```python
from build123d import *

# Parameters (mm, degrees)
SKETCH1_W           = 100
SKETCH1_H           = 110
BOSS_EXTRUDE1_DEPTH = 1.5
CUT_EXTRUDE1_DEPTH  = 10
FILLET1_R           = 4
SKETCH4_R           = 1.6
CUT_EXTRUDE2_DEPTH  = 10


with BuildPart() as part:
    # Sketch1 → Boss-Extrude1 (new body)
    with BuildSketch(Plane(origin=(0, 0, 0), x_dir=(1, 0, 0), z_dir=(0, 1, 0))):
        Rectangle(SKETCH1_W, SKETCH1_H)
    extrude(amount=BOSS_EXTRUDE1_DEPTH)

    # Sketch2 → Cut-Extrude1 (cut)
    with BuildSketch(Plane(origin=(0, 0, 0), x_dir=(-1, 0, 0), z_dir=(0, -1, 0))):
        Polygon((0, 55), (-24, 55), (-24, 3), (24, 3), (24, 55), align=None)
    extrude(amount=-CUT_EXTRUDE1_DEPTH, mode=Mode.SUBTRACT)

    # Fillet1
    fillet1_edges = [part.edges().sort_by_distance(p)[0] for p in [
        (-24, 0.75, -55),
        (-24, 0.75, -3),
        (24, 0.75, -3),
        (24, 0.75, -55),
        (50, 0.75, 55),
        (-50, 0.75, 55),
        (-50, 0.75, -55),
        (50, 0.75, -55),
    ]]
    fillet(fillet1_edges, radius=FILLET1_R)

    # Sketch4 → Cut-Extrude2 (cut)
    with BuildSketch(Plane(origin=(0, 0, 0), x_dir=(-1, 0, 0), z_dir=(0, -1, 0))):
        with Locations((46, -51)):
            Circle(SKETCH4_R)
        with Locations((46, 51)):
            Circle(SKETCH4_R)
        with Locations((-46, 51)):
            Circle(SKETCH4_R)
        with Locations((-46, -51)):
            Circle(SKETCH4_R)
    extrude(amount=-CUT_EXTRUDE2_DEPTH, mode=Mode.SUBTRACT)


solid = part.part
```
Design review of the part built by this model. Coordinates are the model's own, in mm. A direction names the side the tool comes from. Give positions to 0.01 mm unless a question says otherwise; leave off trailing zeros. Write each loop counter-clockwise with the first axis right and the second up, starting at its lowest first coordinate (ties: lowest second). Pieces come first, ordered by that corner, then holes.
(1) Clearance check with a flat-ended pin moving along its axis: pin 1 Ø0.8 at (x, y) = (0.5, 0.5) entering from -Z. State where the tip first meets the part, or that it passes through.
Checked values:
pin 1: stops at z = -3
(2) Add section A-A (z = -25). Give the boundary of the cut face in (x, y).
Checked values:
outline: (-50, 0) - (-24, 0) - (-24, 1.5) - (-50, 1.5) - close; (24, 0) - (50, 0) - (50, 1.5) - (24, 1.5) - close
(3) Mouldability with a two-part tool opening along X and no side actions: class faces 1 (the face through (25.141, 0.76, -53.797)), 2 (the face through (-48.859, 0.76, 53.797)), 3 (the face through (-1, 1.5, 11)), 4 (the face through (48.859, 0.76, -53.797)) as +X half, -X half, draft (parallel to the pull), parting line (faces both ways), or undercut.
Checked values:
face 1: undercut
face 2: -X half
face 3: draft
face 4: +X half
(4) Add section C-C (x = -21.5). Give the boundary of the cut face in (y, z), and give its area (3 significant figures).
Checked values:
outline: (0, -3.29) - (1.5, -3.29) - (1.5, 55) - (0, 55) - close
area: 87.4 mm2
(5) Add section B-B (y = 0.6). Give the boundary of the cut face in (x, z).
Checked values:
outline: (-50, -51) arc R4 ccw to (-46, -55) - (-28, -55) arc R4 ccw to (-24, -51) - (-24, -7) arc R4 cw to (-20, -3) - (20, -3) arc R4 cw to (24, -7) - (24, -51) arc R4 ccw to (28, -55) - (46, -55) arc R4 ccw to (50, -51) - (50, 51) arc R4 ccw to (46, 55) - (-46, 55) arc R4 ccw to (-50, 51) - close; hole circle Ø3.2 at (-46, -51); hole circle Ø3.2 at (-46, 51); hole circle Ø3.2 at (46, -51); hole circle Ø3.2 at (46, 51)
(6) Tool access review of faces 5 (the face through (-1, 0, 11)), 6 (the face through (-25.203, 0.76, -53.859)): name each direction out of +Z, -Z, +X, -X, +Y, -Y from which nothing blocks a thin tool from reaching the whole face with its end or side.
Checked values:
face 5: +Z, -Z, +X, -X, -Y
face 6: -Z, +Y, -Y
(7) Wall thickness on line 1 along X through (y, z) = (0.55, 51); line 2 along Z through (x, y) = (46, 0.85); line 3 along X through (y, z) = (0.75, -51): over which ranges is each line inside the solid? List them lowest first.
Checked values:
line 1: x = -50 to -47.6, -44.4 to 44.4, 47.6 to 50
line 2: z = -55 to -52.6, -49.4 to 49.4, 52.6 to 55
line 3: x = -50 to -47.6, -44.4 to -24, 24 to 44.4, 47.6 to 50
